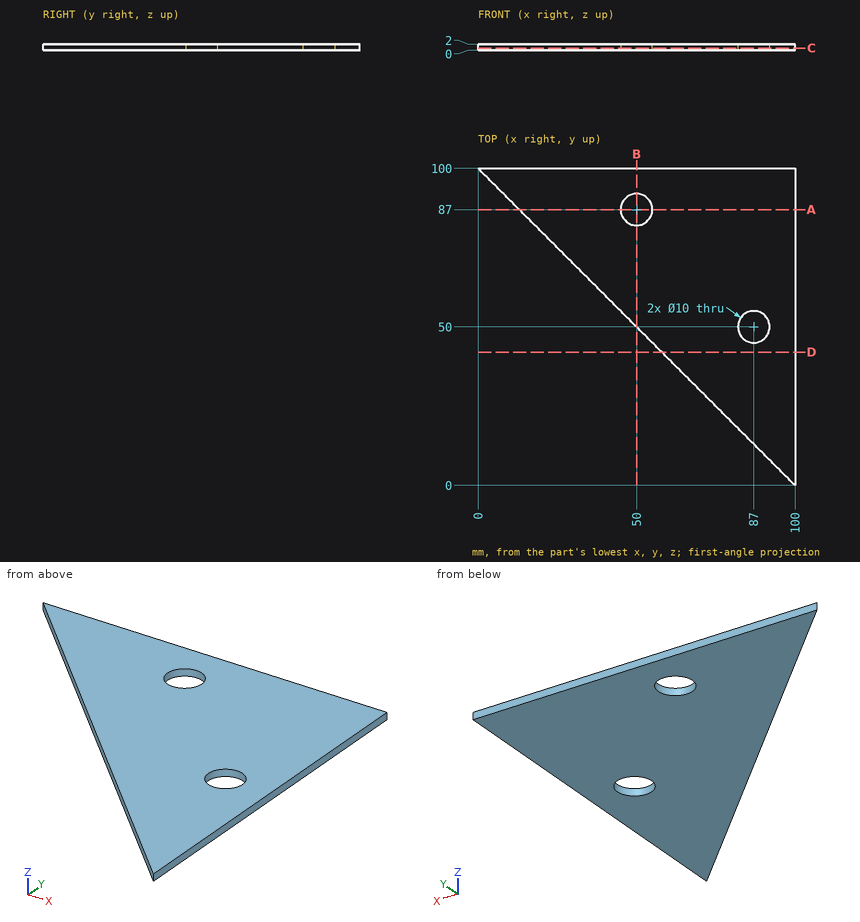
Design review of the part shown in the three views and the two pictorial views. Dimensions are in mm from the part's minimum x, y and z. Round coordinates to 2 decimals unless told otherwise and drop trailing zeros. Loops run counter-clockwise (first coordinate to the right, second up) from the corner with the lowest first, then second, coordinate; pieces in that order, holes last. Notation, with made-up numbers: (15.5, 38.5) - (61.5, 38.5) arc R15 ccw to (61.5, 66.5) - close; hole circle Ø6 at (-30.5, 28.25). An arc over 180 degrees is marked (long way). Use one line per item in the form item = value.
1) We need section D-D on y = 42. Write out the cut boundary in (x, z), then the cut area to 3 significant figures.
Solutions:
outline = (58, 0) - (100, 0) - (100, 2) - (58, 2) - close
area = 84.0 mm2
2) We need section C-C on z = 0.7. Write out the cut boundary in (x, y), then the cut area to 3 significant figures.
Solutions:
outline = (0, 100) - (100, 0) - (100, 100) - close; hole circle Ø10 at (50, 87); hole circle Ø10 at (87, 50)
area = 4,840 mm2
3) We need section B-B on x = 50. Write out the cut boundary in (y, z), then the cut area to 3 significant figures.
Solutions:
outline = (50, 0) - (82, 0) - (82, 2) - (50, 2) - close; (92, 0) - (100, 0) - (100, 2) - (92, 2) - close
area = 80.0 mm2
4) Clearance check with a flat-ended pin moving along its axis: P1, Ø9, axis at x = 87, y = 50, coming from the -Z side. State where the tip first meets the part, or that it passes through.
Solutions:
P1 = through
5) We need section A-A on y = 87. Write out the cut boundary in (x, z), then the cut area to 3 significant figures.
Solutions:
outline = (13, 0) - (45, 0) - (45, 2) - (13, 2) - close; (55, 0) - (100, 0) - (100, 2) - (55, 2) - close
area = 154 mm2
6) Wall thickness on probe 1 along Y at (x, z) = (48, 0.3); probe 2 along Y at (x, z) = (83, 1); probe 3 along Y at (x, z) = (30.5, 1.8): over which ranges is each line inside the solid? List them lowest first.
Solutions:
probe_1 = 52 to 82.42, 91.58 to 100
probe_2 = 17 to 47, 53 to 100
probe_3 = 69.5 to 100
